from build123d import *

# Parameters (mm, degrees)
BOSS_EXTRUDE1_DEPTH = 80
SKETCH2_R           = 2.15
CUT_EXTRUDE1_DEPTH  = 89.328477854
SKETCH3_R           = 2.1
CUT_EXTRUDE2_DEPTH  = 85.835134231
CHAMFER1_SIZE       = 2.3
CHAMFER2_SIZE       = 1


with BuildPart() as part:
    # Sketch1 → Boss-Extrude1 (new body)
    with BuildSketch(Plane.XY):
        Polygon((-10.2, 0), (-10.2, 20.4), (10.2, 20.4), (10.2, 0), (14.2, 0), (14.2, 24.4), (-14.2, 24.4), (-14.2, 0), align=None)
    extrude(amount=BOSS_EXTRUDE1_DEPTH)

    # Sketch2 → Cut-Extrude1 (cut, through all)
    with BuildSketch(Plane(origin=(14.2, 0, 0), x_dir=(0, 0, -1), z_dir=(1, 0, 0))):
        with Locations(Location((-50, 10, 0), (0, 0, 90))):
            Circle(SKETCH2_R)
        with Locations(Location((-70, 10, 0), (0, 0, 90))):
            Circle(SKETCH2_R)
        with Locations(Location((-30, 10, 0), (0, 0, 90))):
            Circle(SKETCH2_R)
        with Locations(Location((-10, 10, 0), (0, 0, 90))):
            Circle(SKETCH2_R)
    extrude(amount=-CUT_EXTRUDE1_DEPTH, mode=Mode.SUBTRACT)

    # Sketch3 → Cut-Extrude2 (cut, through all)
    with BuildSketch(Plane(origin=(0, 24.4, 0), x_dir=(1, 0, 0), z_dir=(0, 1, 0))):
        with Locations(Location((0, -10, 0), (0, 0, 180))):
            Circle(SKETCH3_R)
        with Locations(Location((0, -30, 0), (0, 0, 180))):
            Circle(SKETCH3_R)
        with Locations(Location((0, -50, 0), (0, 0, 180))):
            Circle(SKETCH3_R)
        with Locations(Location((0, -70, 0), (0, 0, 180))):
            Circle(SKETCH3_R)
    extrude(amount=-CUT_EXTRUDE2_DEPTH, mode=Mode.SUBTRACT)

    # Chamfer1
    chamfer1_edges = [part.edges().sort_by_distance(p)[0] for p in [
        (-14.2, 7.85, 10),
        (14.2, 7.85, 10),
        (-14.2, 7.85, 30),
        (14.2, 7.85, 30),
        (-14.2, 7.85, 70),
        (14.2, 7.85, 70),
        (-14.2, 7.85, 50),
        (14.2, 7.85, 50),
        (2.1, 24.4, 10),
        (2.1, 24.4, 30),
        (2.1, 24.4, 50),
        (2.1, 24.4, 70),
    ]]
    chamfer(chamfer1_edges, length=CHAMFER1_SIZE)

    # Chamfer2
    chamfer2_edges = [part.edges().sort_by_distance(p)[0] for p in [
        (-14.2, 0, 40),
        (-14.2, 24.4, 40),
        (14.2, 24.4, 40),
        (14.2, 0, 40),
        (14.2, 12.2, 80),
        (0, 24.4, 80),
        (-14.2, 12.2, 80),
        (-14.2, 12.2, 0),
        (0, 24.4, 0),
        (14.2, 12.2, 0),
    ]]
    chamfer(chamfer2_edges, length=CHAMFER2_SIZE)


solid = part.part
Model file for the job. Use its own axes, mm. A direction names the side the tool comes from. Give positions to 0.01 mm unless a question says otherwise; leave off trailing zeros. Loops run counter-clockwise (first coordinate to the right, second up) from the corner with the lowest first, then second, coordinate; pieces in that order, holes last.
Item 1: Slice it at D-D (z = 20.5). Write the cut outline in (x, y), plus the area to 3 significant figures.
Check values:
outline: (-14.2, 1) - (-13.2, 0) - (-10.2, 0) - (-10.2, 20.4) - (10.2, 20.4) - (10.2, 0) - (13.2, 0) - (14.2, 1) - (14.2, 23.4) - (13.2, 24.4) - (-13.2, 24.4) - (-14.2, 23.4) - close
area: 275 mm2
Item 2: Slice it at C-C (x = -9.25). Write the cut outline in (y, z).
Check values:
outline: (20.4, 0) - (23.4, 0) - (24.4, 1) - (24.4, 79) - (23.4, 80) - (20.4, 80) - close
Item 3: Slice it at A-A (z = 10). Give the number of separate pieces and of enclosed holes in the cut face, plus the area to 3 significant figures.
Check values:
separate pieces: 4
enclosed holes: 0
area: 208 mm2
Item 4: Drill centre lines: line 1 along Z through (x, y) = (11.15, 10); line 2 along X through (y, z) = (15, 64); line 3 along Y through (x, z) = (6.5, 76). Where is each one in solid material? Low to high.
Check values:
line 1: z = 0 to 7.85, 12.15 to 27.85, 32.15 to 47.85, 52.15 to 67.85, 72.15 to 80
line 2: x = -14.2 to -10.2, 10.2 to 14.2
line 3: y = 20.4 to 24.4
Item 5: Mould opens along Y. For faces 1 (the face through (12, 0, 39)), 2 (the face through (-12.044, 9.503, 47.761)), 3 (the face through (-1, 21, 0)) say: +Y half, -Y half, draft (parallel to the pull), parting line (faces both ways), or undercut.
Check values:
face 1: -Y half
face 2: undercut
face 3: draft
Item 6: Drop flat-ended pins along their axis: P1, Ø2.5, axis at y = 10, z = 50, coming from the -X side; P2, Ø1.5, axis at y = 12, z = 70.5, coming from the -X side; P3, Ø5.5, axis at y = 10, z = 50, coming from the +X side; P4, Ø5, axis at x = 3.5, y = 20, coming from the +Z side. Give the stop position or say it passes through.
Check values:
P1: passes through
P2: stops at x = -12.56
P3: stops at x = 12.5
P4: stops at z = 80
Item 7: Which spindle directions (+Z, -Z, +X, -X, +Y, -Y) get a long thin tool onto all of the face, cutting with end or side? Do faces 4 (the face through (0, 24.4, 39)), 5 (the face through (10.2, 10, 39)). Say none if no direction does.
Check values:
face 4: +Z, -Z, +X, -X, +Y
face 5: +Z, -Z, -Y
